Build history of the part. All positions in model axes, mm. A direction names the side the tool comes from. Give positions to 0.01 mm unless a question says otherwise; leave off trailing zeros. Order: outer loops, then holes, each group sorted by start corner. A loop starts at its lowest first (then second) coordinate and runs counter-clockwise, first axis right, second up. Notation, with made-up numbers: M -20,-4 L 32,-4 A22 ccw 32,2 Z; hole C -26.5,78 d7. An arc over 180 degrees is marked long. One line per item, written item: value. Start each with the question number.
from build123d import *

# Parameters (mm, degrees)
F0_R     = 20.6375
F0_R_2   = 17.4625
F1_DEPTH = 381
F2_W     = 41.275
F2_H     = 41.275
F3_DEPTH = 19.05


# Not quite as in the source:
# - a pattern or mirror of a feature is missing from the dataset's text; its kind, count and spacing are read off the source's solid


with BuildPart() as f1:
    # F0 (on Right) → F1 (new body, symmetric)
    with BuildSketch(Plane.YZ):
        Circle(F0_R)
        Circle(F0_R_2, mode=Mode.SUBTRACT)
    extrude(amount=F1_DEPTH, both=True)

    # F2 (on face) → F3 (join)
    with BuildSketch(Plane(origin=(-381, 0, 0), x_dir=(0, -1, 0), z_dir=(-1, 0, 0))):
        Rectangle(F2_W, F2_H)
    f3 = extrude(amount=-F3_DEPTH)

    # F3_copies: F3 across plane
    add(f3.mirror(Plane(origin=(0, 0, 0), x_dir=(0, 0, 1), z_dir=(1, 0, 0))))


solid = f1.part
1) Slice it at A-A (y = -8). List the corners of the cut face in (x, z).
2) Tool access for faces 1 (the flat face through (-361.95, -16, -16)), 2 (the flat face through (361.95, 16, -16)), 3 (the flat face through (361.95, 16, 16)), 4 (the flat face through (361.95, -16, 16)): list every direction of +Z, -Z, +X, -X, +Y, -Y with a clear straight run to the whole face (end or side of a thin tool).
3) Drop flat-ended pins along their axis: P1, Ø2, axis at x = -15, z = 12, coming from the +Y side; P2, Ø6, axis at x = 141.5, z = -7, coming from the +Y side; P3, Ø2, axis at x = -298, y = 12.5, coming from the -Z side. Give the stop position or say it passes through.
4) Slice it at B-B (z = -11). List the corners of the cut face in (x, y), plus the area to 3 significant figures.
5) Drill centre lines: line 1 (Y direction, x = -109, z = 0); line 2 (X direction, y = 2, z = 13.5). Where is each one in solid material? Low to high.
6) Slice it at C-C (x = 125.5). List the corners of the cut face in (y, z) (1 decimal), plus the area to 3 significant figures.
7) Pull direction X, two halves, no side cores. Call faces 5 (the flat face through (381, 0, 0)), 6 (the cylindrical face through (5.067, -4.474, -20.147)), 7 (the flat face through (372, -20.638, 0)), 8 (the flat face through (361.95, -16, -16)): pulls with the +X half, pulls with the -X half, needs draft (parallel to the pull), parting line crosses it, or undercut.
Results list:
1. outline: M -381,-20.64 L -361.95,-20.64 L -361.95,-19.02 L 361.95,-19.02 L 361.95,-20.64 L 381,-20.64 L 381,20.64 L 361.95,20.64 L 361.95,19.02 L -361.95,19.02 L -361.95,20.64 L -381,20.64 Z; hole M -361.95,-15.52 L 361.95,-15.52 L 361.95,15.52 L -361.95,15.52 Z
2. face 1: -Z, -Y
2. face 2: -Z, +Y
2. face 3: +Z, +Y
2. face 4: +Z, -Y
3. P1: stops at y = 17.46
3. P2: stops at y = 20.25
3. P3: stops at z = -17.14
4. outline: M -381,-20.64 L -361.95,-20.64 L -361.95,-17.46 L 361.95,-17.46 L 361.95,-20.64 L 381,-20.64 L 381,20.64 L 361.95,20.64 L 361.95,17.46 L -361.95,17.46 L -361.95,20.64 L -381,20.64 Z; hole M -361.95,-13.56 L 361.95,-13.56 L 361.95,13.56 L -361.95,13.56 Z
4. area: 7,220 mm²
5. line 1: y = -20.64 to -17.46, 17.46 to 20.64
5. line 2: x = -381 to -361.95, 361.95 to 381
6. outline: C 0,0 d41.3; hole C 0,0 d34.9
6. area: 380 mm²
7. face 5: pulls with the +X half
7. face 6: undercut
7. face 7: needs draft
7. face 8: undercut
